```python
from build123d import *

# Parameters (mm, degrees)
CYLINDER006_R     = 1.6
CYLINDER006_DEPTH = 10
CYLINDER007_R     = 1.6
CYLINDER007_DEPTH = 10
CYLINDER004_R     = 6.2
CYLINDER004_DEPTH = 10
BOX002_W          = 5.4
BOX002_H          = 5
BOX002_DEPTH      = 2
CYLINDER005_R     = 1.6
CYLINDER005_DEPTH = 10
CYLINDER001_R     = 2.1
CYLINDER001_DEPTH = 10
CYLINDER_R        = 2.1
CYLINDER_DEPTH    = 10
CYLINDER002_R     = 2.1
CYLINDER002_DEPTH = 10
CYLINDER003_R     = 2.1
CYLINDER003_DEPTH = 10
BOX_W             = 45.2
BOX_H             = 20
BOX_DEPTH         = 2
BOX001_W          = 5.4
BOX001_H          = 5
BOX001_DEPTH      = 2


with BuildPart() as cylinder006:
    # Cylinder006 → Cylinder006 (new body)
    with BuildSketch(Plane(origin=(14.75, 22.5, -4), x_dir=(1, 0, 0), z_dir=(0, 0, 1))):
        Circle(CYLINDER006_R)
    extrude(amount=CYLINDER006_DEPTH)


with BuildPart() as cylinder007:
    # Cylinder007 → Cylinder007 (new body)
    with BuildSketch(Plane(origin=(14.75, -2.5, -4), x_dir=(1, 0, 0), z_dir=(0, 0, 1))):
        Circle(CYLINDER007_R)
    extrude(amount=CYLINDER007_DEPTH)


with BuildPart() as cylinder004:
    # Cylinder004 → Cylinder004 (new body)
    with BuildSketch(Plane(origin=(14.75, 10, -4), x_dir=(1, 0, 0), z_dir=(0, 0, 1))):
        Circle(CYLINDER004_R)
    extrude(amount=CYLINDER004_DEPTH)


with BuildPart() as cube001:
    # Box002 → Box002 (new body)
    with BuildSketch(Plane(origin=(12.05, 20, 0), x_dir=(1, 0, 0), z_dir=(0, 0, 1))):
        with Locations((2.7, 2.5)):
            Rectangle(BOX002_W, BOX002_H)
    extrude(amount=BOX002_DEPTH)


with BuildPart() as cylinder005:
    # Cylinder005 → Cylinder005 (new body)
    with BuildSketch(Plane(origin=(30.45, 10, -5), x_dir=(1, 0, 0), z_dir=(0, 0, 1))):
        Circle(CYLINDER005_R)
    extrude(amount=CYLINDER005_DEPTH)


with BuildPart() as cylinder001:
    # Cylinder001 → Cylinder001 (new body)
    with BuildSketch(Plane(origin=(41.95, 3.25, -5), x_dir=(1, 0, 0), z_dir=(0, 0, 1))):
        Circle(CYLINDER001_R)
    extrude(amount=CYLINDER001_DEPTH)


with BuildPart() as cylinder:
    # Cylinder → Cylinder (new body)
    with BuildSketch(Plane(origin=(41.95, 16.75, -5), x_dir=(1, 0, 0), z_dir=(0, 0, 1))):
        Circle(CYLINDER_R)
    extrude(amount=CYLINDER_DEPTH)


with BuildPart() as cylinder002:
    # Cylinder002 → Cylinder002 (new body)
    with BuildSketch(Plane(origin=(3.25, 16.75, -5), x_dir=(1, 0, 0), z_dir=(0, 0, 1))):
        Circle(CYLINDER002_R)
    extrude(amount=CYLINDER002_DEPTH)


with BuildPart() as cylinder003:
    # Cylinder003 → Cylinder003 (new body)
    with BuildSketch(Plane(origin=(3.25, 3.25, -5), x_dir=(1, 0, 0), z_dir=(0, 0, 1))):
        Circle(CYLINDER003_R)
    extrude(amount=CYLINDER003_DEPTH)


with BuildPart() as fusion:
    # Box → Box (new body)
    with BuildSketch(Plane.XY):
        with Locations((22.6, 10)):
            Rectangle(BOX_W, BOX_H)
    extrude(amount=BOX_DEPTH)

    # Cut: cut Cylinder003
    add(cylinder003.part, mode=Mode.SUBTRACT)

    # Cut001: cut Cylinder002
    add(cylinder002.part, mode=Mode.SUBTRACT)

    # Cut002: cut Cylinder
    add(cylinder.part, mode=Mode.SUBTRACT)

    # Cut003: cut Cylinder001
    add(cylinder001.part, mode=Mode.SUBTRACT)

    # Cut004: cut Cylinder004
    add(cylinder004.part, mode=Mode.SUBTRACT)

    # Cut005: cut Cylinder005
    add(cylinder005.part, mode=Mode.SUBTRACT)

    # Fusion: union Cube001
    add(cube001.part)


with BuildPart() as cut008:
    # Box001 → Box001 (new body)
    with BuildSketch(Plane(origin=(12.05, -5, 0), x_dir=(1, 0, 0), z_dir=(0, 0, 1))):
        with Locations((2.7, 2.5)):
            Rectangle(BOX001_W, BOX001_H)
    extrude(amount=BOX001_DEPTH)

    # Fusion001: union Fusion
    add(fusion.part)

    # Cut006: cut Cylinder004
    add(cylinder004.part, mode=Mode.SUBTRACT)

    # Cut007: cut Cylinder007
    add(cylinder007.part, mode=Mode.SUBTRACT)

    # Cut008: cut Cylinder006
    add(cylinder006.part, mode=Mode.SUBTRACT)


solid = cut008.part
```
For this review, take the finished solid that the model builds, in its own axes (mm). A direction names the side the tool comes from. Coordinates: 2 decimals unless noted, no trailing zeros. Write each loop counter-clockwise with the first axis right and the second up, starting at its lowest first coordinate (ties: lowest second). Pieces come first, ordered by that corner, then holes.
(1) Add section B-B on y = -2.5. Give the boundary of the cut face in (x, z), then the cut area to 3 significant figures.
(2) The part is to be moulded in two halves that separate along Y. For faces 1 (the face through (6, 20, 1)), 2 (the face through (6, 0, 1)), 3 (the face through (13.406, 3.947, 0.986)), say which applies: +Y half, -Y half, draft (parallel to the pull), parting line (faces both ways), or undercut.
(3) For pin 1 Ø0.6 at (y, z) = (22, 1) entering from -X; pin 2 Ø1 at (y, z) = (22, 1) entering from +X, all flat-tipped, find the tip position at first contact; note any pin that passes through.
(4) Tool access review of faces 4 (the face through (31, 0, 1)), 5 (the face through (12.05, 22, 1)), 6 (the face through (12.05, -3, 1)), 7 (the face through (17.45, 22, 1)): name each direction out of +Z, -Z, +X, -X, +Y, -Y from which nothing blocks a thin tool from reaching the whole face with its end or side.
(5) Add section D-D on y = 16.75. Give the boundary of the cut face in (x, z), then the cut area to 3 significant figures.
(6) Add section A-A on x = 14.75. Give the boundary of the cut face in (y, z), then the cut area to 3 significant figures.
(7) Wall thickness on probe 1 along Y at (x, z) = (14.75, 1.45); probe 2 along Y at (x, z) = (3.25, 1.25); probe 3 along X at (y, z) = (16.75, 0.55): over which ranges is each line inside the solid? List them lowest first.
(8) Add section C-C on z = 0.6. Count the separate pieces of the cut face and the enclosed holes in it, then the cut area to 3 significant figures.
Answer sheet:
1. outline: (12.05, 0) - (13.15, 0) - (13.15, 2) - (12.05, 2) - close; (16.35, 0) - (17.45, 0) - (17.45, 2) - (16.35, 2) - close
1. area: 4.40 mm2
2. face 1: +Y half
2. face 2: -Y half
2. face 3: undercut
3. pin 1: stops at x = 12.05
3. pin 2: stops at x = 17.45
4. face 4: +Z, -Z, +X, -Y
4. face 5: +Z, -Z, -X, +Y
4. face 6: +Z, -Z, -X, -Y
4. face 7: +Z, -Z, +X, +Y
5. outline: (0, 0) - (1.15, 0) - (1.15, 2) - (0, 2) - close; (5.35, 0) - (39.85, 0) - (39.85, 2) - (5.35, 2) - close; (44.05, 0) - (45.2, 0) - (45.2, 2) - (44.05, 2) - close
5. area: 73.6 mm2
6. outline: (-5, 0) - (-4.1, 0) - (-4.1, 2) - (-5, 2) - close; (-0.9, 0) - (3.8, 0) - (3.8, 2) - (-0.9, 2) - close; (16.2, 0) - (20.9, 0) - (20.9, 2) - (16.2, 2) - close; (24.1, 0) - (25, 0) - (25, 2) - (24.1, 2) - close
6. area: 22.4 mm2
7. probe 1: y = -5 to -4.1, -0.9 to 3.8, 16.2 to 20.9, 24.1 to 25
7. probe 2: y = 0 to 1.15, 5.35 to 14.65, 18.85 to 20
7. probe 3: x = 0 to 1.15, 5.35 to 39.85, 44.05 to 45.2
8. separate pieces: 1
8. enclosed holes: 8
8. area: 758 mm2
